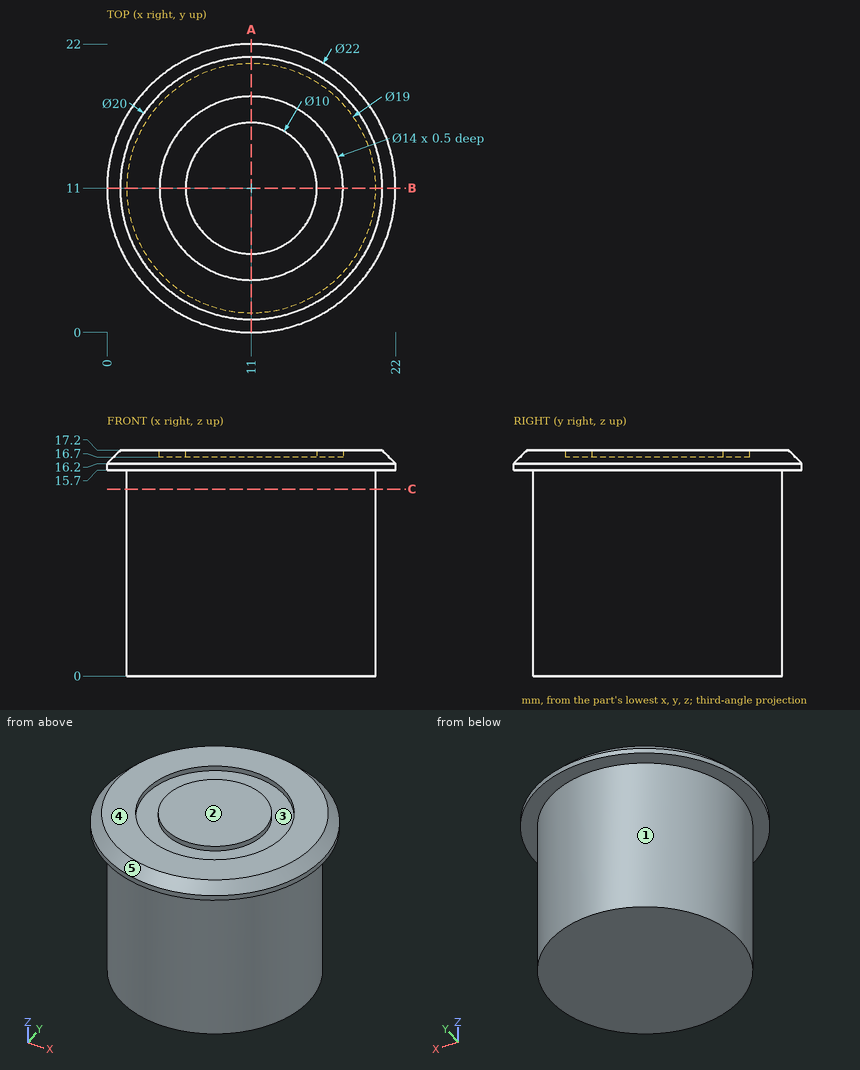
The drawing under review shows one solid part. Ordinate dimensions are in mm from its lowest x, y, z. A direction names the side the tool comes from. Coordinates: 2 decimals unless noted, no trailing zeros. Order: outer loops, then holes, each group sorted by start corner. A loop starts at its lowest first (then second) coordinate and runs counter-clockwise, first axis right, second up. Notation, with made-up numbers: M 28,47.25 L 72,47.25 A20 ccw 72,61.25 Z; hole C 38,38.5 d3. An arc over 180 degrees is marked long. One line per question, with ' | ' between items.
(1) Machinability: for the marked faces 1 and 2, which of the approach directions +Z, -Z, +X, -X, +Y, -Y give a long, thin tool a straight path to every point of the face, cutting with its end or side? Answer none if there is none.
Geometry results:
face 1: -Z | face 2: +Z, +X, -X, +Y, -Y
(2) Add section A-A, the plane x = 11. Write out the cut boundary in (y, z), then the cut area to 3 significant figures.
Geometry results:
outline: M 0,15.7 L 1.5,15.7 L 1.5,0 L 20.5,0 L 20.5,15.7 L 22,15.7 L 22,16.2 L 21,17.2 L 18,17.2 L 18,16.7 L 16,16.7 L 16,17.2 L 6,17.2 L 6,16.7 L 4,16.7 L 4,17.2 L 1,17.2 L 0,16.2 Z | area: 328 mm²
(3) Add section C-C, the plane z = 14.25. Write out the cut boundary in (x, y), then the cut area to 3 significant figures.
Geometry results:
outline: C 11,11 d19 | area: 284 mm²
(4) The part is to be moulded in two halves that separate along X. For the marked faces 3, 4 and 5, say which applies: +X half, -X half, draft (parallel to the pull), parting line (faces both ways), or undercut.
Geometry results:
face 3: undercut | face 4: draft | face 5: parting line
(5) Insertion check: pin 1 (2 mm diameter, centred on y = 3, z = 5.5, fed in from -X); pin 2 (1.5 mm diameter, centred on x = 17.5, z = 15.5, fed in from -Y); pin 3 (4 mm diameter, centred on x = 18, y = 9, fed in from -Z); pin 4 (2 mm diameter, centred on y = 17.5, z = 8, fed in from +X). Each pin has a flat end and moves straight along its axis. Give the tip position at first contact, or say it passes through.
Geometry results:
pin 1: stops at x = 4.58 | pin 2: stops at y = 1.64 | pin 3: stops at z = 0 | pin 4: stops at x = 18.75
(6) For probe 1 along Y at (x, z) = (11, 16.95); probe 2 along Y at (x, z) = (11, 16.9); probe 3 along Z at (x, y) = (6, 8.75), list the stretches that pass through material, from the lowest coordinate up. Write a range as from..to.
Geometry results:
probe 1: y = 0.75..4, 6..16, 18..21.25 | probe 2: y = 0.7..4, 6..16, 18..21.3 | probe 3: z = 0..16.7
